```python
from build123d import *

# Parameters (mm, degrees)
F0_W     = 50
F0_H     = 9
F1_DEPTH = 6
F2_R     = 3
F3_DEPTH = 25
F4_R     = 2.5
F5_DEPTH = 2


with BuildPart() as f1:
    # F0 (on Front) → F1 (new body)
    with BuildSketch(Plane.XZ):
        with Locations((25, 4.5)):
            Rectangle(F0_W, F0_H)
    extrude(amount=F1_DEPTH)

    # F2 (on face) → F3 (cut)
    with BuildSketch(Plane.XZ.offset(6)):
        with Locations((4, 4.2)):
            Circle(F2_R)
        with Locations((11, 4.2)):
            Circle(F2_R)
        with Locations((18, 4.2)):
            Circle(F2_R)
        with Locations((25, 4.2)):
            Circle(F2_R)
        with Locations((32, 4.2)):
            Circle(F2_R)
        with Locations((39, 4.2)):
            Circle(F2_R)
        with Locations((46, 4.2)):
            Circle(F2_R)
    extrude(amount=-F3_DEPTH, mode=Mode.SUBTRACT)

    # F4 (on face) → F5 (join)
    with BuildSketch(Plane.XY.offset(9)):
        with Locations((4, -3)):
            Circle(F4_R)
        with Locations((11, -3)):
            Circle(F4_R)
        with Locations((18, -3)):
            Circle(F4_R)
        with BuildLine():
            ThreePointArc((27.5, -3), (26.767766953, -1.232233047), (25, -0.5))
            Line((25, -0.5), (25, -5.5))
            ThreePointArc((25, -5.5), (26.767766953, -4.767766953), (27.5, -3))
        make_face()
        with BuildLine():
            Line((25, -5.5), (25, -0.5))
            ThreePointArc((25, -0.5), (22.5, -3), (25, -5.5))
        make_face()
        with Locations((32, -3)):
            Circle(F4_R)
        with Locations((39, -3)):
            Circle(F4_R)
        with Locations((46, -3)):
            Circle(F4_R)
    extrude(amount=F5_DEPTH)


solid = f1.part
```
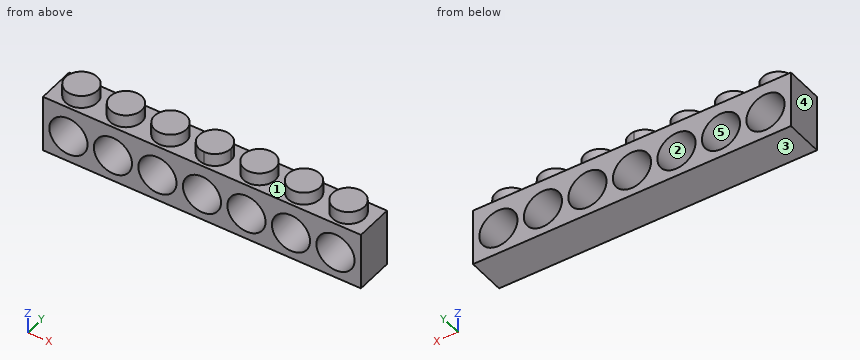
Verification items for the finished model (mm, model axes). Face numbers are marked on the shaded views. A direction names the side the tool comes from. Coordinates: 2 decimals unless noted, no trailing zeros. Write each loop counter-clockwise with the first axis right and the second up, starting at its lowest first coordinate (ties: lowest second). Pieces come first, ordered by that corner, then holes. Notation, with made-up numbers: (38.25, 6.5) - (63.25, 6.5) arc R11 cw to (63.25, 19.5) - close; hole circle Ø6 at (-13, -10). An arc over 180 degrees is marked (long way). One line per question, with ' | ' between items. Start each with the question number.
1. Section check B-B (z = 9.5). Enter the section's corners in (x, y), plus the area to 3 significant figures.
2. Draft check along X on the marked faces 3, 4 and 5. Enter one of: released by +X, released by -X, zero draft, split by the parting line, or undercut.
3. Section check D-D (x = 37). Enter the section's corners in (y, z).
4. Material ranges on line 1 along Z through (x, y) = (4, -1.35); line 2 along Z through (x, y) = (46, -0.35), recorded low to high.
5. Section check A-A (x = 11). Enter the section's corners in (y, z), plus the area to 3 significant figures.
6. Access from +Z, -Z, +X, -X, +Y, -Y to the whole of each face (thin tool, end or side, straight path). Record for the marked faces 1 and 2.
7. Section check C-C (z = 3.5). Count the separate pieces of the cut face and the enclosed holes in it, plus the area to 3 significant figures.
Computed values:
1) outline: circle Ø5 at (4, -3); circle Ø5 at (11, -3); circle Ø5 at (18, -3); circle Ø5 at (25, -3); circle Ø5 at (32, -3); circle Ø5 at (39, -3); circle Ø5 at (46, -3) | area: 137 mm²
2) face 3: zero draft | face 4: released by -X | face 5: undercut
3) outline: (-6, 0) - (0, 0) - (0, 1.96) - (-6, 1.96) - close; (-6, 6.44) - (0, 6.44) - (0, 9) - (-1.5, 9) - (-1.5, 11) - (-4.5, 11) - (-4.5, 9) - (-6, 9) - close
4) line 1: 0 to 1.2, 7.2 to 11 | line 2: 0 to 1.2, 7.2 to 9
5) outline: (-6, 0) - (0, 0) - (0, 1.2) - (-6, 1.2) - close; (-6, 7.2) - (0, 7.2) - (0, 9) - (-0.5, 9) - (-0.5, 11) - (-5.5, 11) - (-5.5, 9) - (-6, 9) - close | area: 28.0 mm²
6) face 1: +Z | face 2: +Y, -Y
7) separate pieces: 8 | enclosed holes: 0 | area: 55.0 mm²
